The listing builds one solid part. Answer for the finished solid, in the listing's coordinates (mm). Face numbers are marked on the shaded views. Give positions to 0.01 mm unless a question says otherwise; leave off trailing zeros. Loops run counter-clockwise (first coordinate to the right, second up) from the corner with the lowest first, then second, coordinate; pieces in that order, holes last.
Item 1: Section D-D, the plane x = 0 is taken. Give the vertices of the cut face in (y, z).
Item 2: Section C-C, the plane y = 0 is taken. Give the vertices of the cut face in (x, z), and give its area (3 significant figures).
Item 3: Each of these flat-tipped pins is pushed along its axis until it touches: pin 1 Ø7 at (y, z) = (0, 90) entering from +X; pin 2 Ø2 at (y, z) = (-6, 198.5) entering from +X; pin 3 Ø9 at (x, z) = (0, 90) entering from -Y. Where does it stop, or does it pass through?
Item 4: The mould has two halves that part along X. Classify the marked faces 1, 2 and 3: pulls with the +X half, pulls with the -X half, needs draft (parallel to the pull), parting line crosses it, or undercut.
Item 5: Section B-B, the plane z = 90 is taken. Give the vertices of the cut face in (x, y).
Item 6: Section A-A, the plane x = 13 is taken. Give the vertices of the cut face in (y, z).
Item 7: Consider line 1 along X through (y, z) = (-28, 240.5); line 2 along X through (y, z) = (39, 90); line 3 along Y through (x, z) = (-9, 341). Determine where each line is inside the solid, lowest interval first.
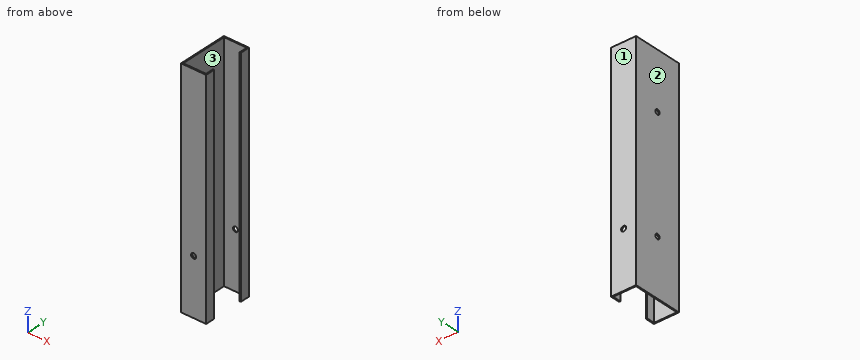
from build123d import *

# Parameters (mm, degrees)
SALIENTE_EXTRUIR1_DEPTH = 360
CROQUIS2_R              = 4
CORTAR_EXTRUIR1_DEPTH   = 365.417343166
CROQUIS3_R              = 4
CORTAR_EXTRUIR2_DEPTH   = 370.323706252


with BuildPart() as part:
    # Croquis1 → Saliente-Extruir1 (new body)
    with BuildSketch(Plane.XY):
        Polygon((18.1, -38.1), (18.1, -25), (20, -25), (20, -38.1), (20, -40), (-20, -40), (-20, 40), (20, 40), (20, 25), (18.1, 25), (18.1, 38.1), (-18.1, 38.1), (-18.1, -38.1), align=None)
    extrude(amount=SALIENTE_EXTRUIR1_DEPTH)

    # Croquis2 → Cortar-Extruir1 (cut, through all)
    with BuildSketch(Plane.ZY.offset(20)):
        with Locations((270, 0)):
            Circle(CROQUIS2_R)
        with Locations((90, 0)):
            Circle(CROQUIS2_R)
    extrude(amount=-CORTAR_EXTRUIR1_DEPTH, mode=Mode.SUBTRACT)

    # Croquis3 → Cortar-Extruir2 (cut, through all)
    with BuildSketch(Plane(origin=(0, 40, 0), x_dir=(1, 0, 0), z_dir=(0, 1, 0))):
        with Locations(Location((0, -90, 0), (0, 0, 270))):
            Circle(CROQUIS3_R)
    extrude(amount=-CORTAR_EXTRUIR2_DEPTH, mode=Mode.SUBTRACT)


solid = part.part
Worked answers:
1. outline: (-40, 0) - (-38.1, 0) - (-38.1, 86) - (-40, 86) - close; (-40, 94) - (-38.1, 94) - (-38.1, 360) - (-40, 360) - close; (38.1, 0) - (40, 0) - (40, 86) - (38.1, 86) - close; (38.1, 94) - (40, 94) - (40, 360) - (38.1, 360) - close
2. outline: (-20, 0) - (-18.1, 0) - (-18.1, 86) - (-20, 86) - close; (-20, 94) - (-18.1, 94) - (-18.1, 266) - (-20, 266) - close; (-20, 274) - (-18.1, 274) - (-18.1, 360) - (-20, 360) - close
2. area: 654 mm2
3. pin 1: passes through
3. pin 2: stops at x = -18.1
3. pin 3: stops at y = -40
4. face 1: needs draft
4. face 2: pulls with the -X half
4. face 3: undercut
5. outline: (-20, -40) - (-4, -40) - (-4, -38.1) - (-18.1, -38.1) - (-18.1, -4) - (-20, -4) - close; (-20, 4) - (-18.1, 4) - (-18.1, 38.1) - (-4, 38.1) - (-4, 40) - (-20, 40) - close; (4, -40) - (20, -40) - (20, -25) - (18.1, -25) - (18.1, -38.1) - (4, -38.1) - close; (4, 38.1) - (18.1, 38.1) - (18.1, 25) - (20, 25) - (20, 40) - (4, 40) - close
6. outline: (-40, 0) - (-38.1, 0) - (-38.1, 360) - (-40, 360) - close; (38.1, 0) - (40, 0) - (40, 360) - (38.1, 360) - close
7. line 1: x = -20 to -18.1, 18.1 to 20
7. line 2: x = -20 to -4, 4 to 20
7. line 3: y = -40 to -38.1, 38.1 to 40
